Check sheet for the modelled part. Datum: model origin and axes. Units: mm. A direction names the side the tool comes from. Round coordinates to 2 decimals unless told otherwise and drop trailing zeros. Write each loop counter-clockwise with the first axis right and the second up, starting at its lowest first coordinate (ties: lowest second). Pieces come first, ordered by that corner, then holes. Notation, with made-up numbers: (-20, -15) - (11, -15) arc R35 ccw to (11, 21) - close; hole circle Ø3 at (47, 80). An arc over 180 degrees is marked (long way). Answer as a JSON object with one key per item and string values. Group by question number.
Item 1: Gauge pin test, flat ends, axial feed: P1, Ø14, axis at y = -9, z = 10, coming from the +X side; P2, Ø4, axis at x = 35, y = -31.5, coming from the -Z side; P3, Ø2.5, axis at y = 31, z = -1.5, coming from the +X side. Record the tip position at first contact, or that the pin passes through.
Item 2: Set-up check for faces 5 (the flat face through (24, 13, 32)), 6 (the flat face through (1, 0, 0)), 7 (the flat face through (14.5, 13, 32)), 8 (the flat face through (35, 4, 31)), 9 (the flat face through (34, -31, -4)): record each of +Z, -Z, +X, -X, +Y, -Y from which the full face is reachable in a straight line by a thin tool's end or side.
Item 3: Release check for a two-part mould opening along Z. For faces 1 (the flat face through (34, 31, -4)), 2 (the flat face through (0, 26, 26)), 3 (the flat face through (34, 31, 4)), 4 (the cylindrical face through (19.316, -35.694, -4.686)) record: pulls with the +Z half, pulls with the -Z half, needs draft (parallel to the pull), parting line crosses it, or undercut.
Item 4: Sectioned sample at D-D on x = 26. Record the boundary of the cut face in (y, z).
Item 5: Thickness scan on line 1 (X direction, y = -48.5, z = 27); line 2 (Z direction, x = 26.5, y = 0); line 3 (X direction, y = 8, z = -4). Record the ranges inside material, lowest first.
Item 6: Sectioned sample at C-C on z = 0. Record the boundary of the cut face in (x, y).
Item 7: Sectioned sample at A-A on x = 34.5. Record the boundary of the cut face in (y, z), plus the area to 3 significant figures.
Item 8: Sectioned sample at B-B on y = 0. Record the boundary of the cut face in (x, z), plus the area to 3 significant figures.
Autodesk Inventor part; units mm, degrees
ref_plane "YZ Plane" through (0, 0, 0) normal (1, 0, 0) x (0, 1, 0)
ref_plane "XZ Plane" through (0, 0, 0) normal (0, 1, 0) x (-1, 0, 0)
ref_plane "XY Plane" through (0, 0, 0) normal (0, 0, 1) x (1, 0, 0)
sketch "草图1" plane through (0, 0, 0) normal (0, 1, 0) x (-1, 0, 0)
  line L0 (0, 61) -> (-12, 61)
  line L1 (-12, 61) -> (-12, 34)
  line L2 (-12, 34) -> (-14.5, 34)
  line L3 (-14.5, 34) -> (-14.5, 36)
  line L4 (-14.5, 36) -> (-24, 36)
  line L5 (-24, 36) -> (-24, 34)
  line L6 (-24, 34) -> (-38, 34)
  line L7 (-38, 34) -> (-38, 0)
  line L8 (-38, 0) -> (0, 0)
  line L9 (0, 0) -> (0, 61)
  line L10 (0, 34) -> (-1, 33)
  line L11 (-1, 33) -> (-1, 0)
  line L12 (-38, 30) -> (-15, 27.6998)
  line L13 (-15, 27.6998) -> (-15, 0)
  line L14 (7.6, 0) -> (-45.6, 0)
  dimension "d2" = 61
  dimension "d4" = 26
  dimension "d5" = 12
  dimension "d6" = 36
  dimension "d7" = 34
  dimension "d8" = 12
  dimension "d9" = 2.5
  dimension "d10" = 34
  dimension "d11" = 45
  dimension "d12" = 1
  dimension "d13" = 15
  dimension "d14" = 30
  dimension "d15" = 84.289
revolve "旋转1" add sketch "草图1" angle 360 about axis through (-10, 0, 0) along (1, 0, 0) contours L9 L10 L11 L8 L13 L12 L7 L6 L5 L4 L3 L2 L1 L0
sketch "草图2" plane through (0, 0, 0) normal (0, 1, 0) x (-1, 0, 0)
  line L0 (-24, 34) -> (-38, 34)
  line L1 (-38, 34) -> (-31, 34)
  line L2 (-31, 34) -> (-31, -24)
  line L3 (-31, -24) -> (-38, -24)
  line L4 (-38, -24) -> (-38, 34)
  point P0 (0, 0)
  dimension "d17" = 7
extrude "拉伸1" cut sketch "草图2" along normal mid plane 8
sketch "草图3" plane through (0, 0, 0) normal (0, 0, 1) x (1, 0, 0)
  line L0 (38, 4) -> (38, 34)
  line L1 (24, -34) -> (38, -34)
  line L2 (38, 34) -> (31, 34)
  line L3 (31, 34) -> (31, -34)
  line L4 (31, -34) -> (38, -34)
  line L5 (38, -34) -> (38, 34)
  point P0 (0, 0)
  point P1 (38, -4)
  dimension "d20" = 7
extrude "拉伸2" cut sketch "草图3" along normal mid plane 8
sketch "草图4" plane through (0, 0, 0) normal (-1, 0, 0) x (0, 0, 1)
  circle A0 centre (34.2947, 34.2947) radius 5.5
  circle A1 centre (-34.2947, 34.2947) radius 5.5
  circle A2 centre (-34.2947, -34.2947) radius 5.5
  circle A3 centre (34.2947, -34.2947) radius 5.5
  line L0 (34.2947, 34.2947) -> (0, 0)
  line L1 (0, -85.4) -> (0, 85.4)
  dimension "d23" = 11
  dimension "d24" = 48.5
  dimension "d27" = 360
  dimension "d35" = 45
extrude "拉伸3" cut sketch "草图4" against normal up to surface (12 mm away)
chamfer "倒角1" distance 1 angle 45 1 edges at (0, 0, -61)
fillet "圆角1" radius 5 1 edges at (15, 0, -27.6998)
equation "\"d2\" = 0.5 * D2"
equation "\"d4\" = M"
equation "\"d5\" = e"
equation "\"d6\" = 0.5 * D"
equation "\"d7\" = 0.5 * D_d"
equation "\"d8\" = e1"
equation "\"d10\" = 0.5 * D_d"
equation "\"d13\" = b1"
equation "\"d14\" = 0.5 * D4"
equation "\"d17\" = h_b"
equation "\"d18\" = b"
equation "\"d20\" = h_b"
equation "\"d21\" = b"
equation "\"d23\" = d0"
equation "\"d24\" = 0.5 * D0"
equation "\"d29\" = b"
equation "\"d0\" = 11"
equation "\"D\" = 72"
equation "\"D0\" = 97"
equation "\"D2\" = 122"
equation "\"D_d\" = 68"
equation "\"e\" = 12"
equation "\"e1\" = 12"
equation "\"b\" = 8"
equation "\"h_b\" = 7"
equation "\"M\" = 26"
equation "\"b1\" = 15"
equation "\"d1\" = 26"
properties part number "中间轴承闷盖" material "灰口铁"
Completed:
{
 "1": {"P1": "x = 15", "P2": "z = -16.9", "P3": "x = 31"},
 "2": {"face 5": "+X", "face 6": "-X", "face 7": "none", "face 8": "+Z, +X", "face 9": "+X, +Y, -Y"},
 "3": {"face 1": "undercut", "face 2": "needs draft", "face 3": "undercut", "face 4": "parting line crosses it"},
 "4": {"outline": "circle Ø68 at (0, 0); hole circle Ø57.6 at (0, 0)"},
 "5": {"line 1": "0 to 12", "line 2": "-34 to -28.85, 28.85 to 34", "line 3": "1 to 15"},
 "6": {"outline": "(0, -60) - (1, -61) - (12, -61) - (12, -34) - (14.5, -34) - (14.5, -36) - (24, -36) - (24, -34) - (31, -34) - (31, -29.3) - (19.5, -28.15) arc R5 cw to (15, -23.17) - (15, 23.17) arc R5 cw to (19.5, 28.15) - (31, 29.3) - (31, 34) - (24, 34) - (24, 36) - (14.5, 36) - (14.5, 34) - (12, 34) - (12, 61) - (1, 61) - (0, 60) - (0, 34) - (1, 33) - (1, -33) - (0, -34) - close"},
 "7": {"outline": "(-33.76, -4) arc R34 ccw to (33.76, -4) - (29.38, -4) arc R29.65 cw to (-29.38, -4) - close; (-33.76, 4) - (-29.38, 4) arc R29.65 cw to (-4, 29.38) - (-4, 33.76) arc R34 ccw to start; (4, 29.38) arc R29.65 cw to (29.38, 4) - (33.76, 4) arc R34 ccw to (4, 33.76) - close", "area": "765 mm²"},
 "8": {"outline": "(0, -60) - (1, -61) - (12, -61) - (12, -34) - (14.5, -34) - (14.5, -36) - (24, -36) - (24, -34) - (38, -34) - (38, -30) - (19.5, -28.15) arc R5 cw to (15, -23.17) - (15, 23.17) arc R5 cw to (19.5, 28.15) - (31, 29.3) - (31, 34) - (24, 34) - (24, 36) - (14.5, 36) - (14.5, 34) - (12, 34) - (12, 61) - (1, 61) - (0, 60) - (0, 34) - (1, 33) - (1, -33) - (0, -34) - close", "area": "1,850 mm²"}
}
